Geometry check sheet. Reference: the model listing, model coordinates, mm. Face numbers are marked on the shaded views. A direction names the side the tool comes from. Give positions to 0.01 mm unless a question says otherwise; leave off trailing zeros. Order: outer loops, then holes, each group sorted by start corner. A loop starts at its lowest first (then second) coordinate and runs counter-clockwise, first axis right, second up. Notation, with made-up numbers: M 64,81.25 L 71,81.25 A25 cw 71,94.25 Z; hole C 29.5,-35.5 d2. An arc over 180 degrees is marked long. Answer as a JSON object with one key per item and string values. Group by question number.
Autodesk Inventor part; units mm, degrees
ref_plane "YZ Plane" through (0, 0, 0) normal (1, 0, 0) x (0, 1, 0)
ref_plane "XZ Plane" through (0, 0, 0) normal (0, 1, 0) x (-1, 0, 0)
ref_plane "XY Plane" through (0, 0, 0) normal (0, 0, 1) x (1, 0, 0)
ref_plane "РабПлоскость1" through (-45, 39.0097, 0) normal (-0.9659258, 0, 0.258819) x (0, -1, 0)
sketch "Эскиз1" plane through (-45, 39.0097, 0) normal (-0.9659258, 0, 0.258819) x (0, -1, 0)
  line L0 (0, 0) -> (78.0194, 0)
  line L1 (0.0194, 85.4597) -> (78.0194, 85.4597)
  line L2 (78.0194, 68.8953) -> (78.0194, 85.4597)
  line L3 (-2.9723, 68.8953) -> (78.0194, 68.8953)
  line L4 (-2.9723, 68.8953) -> (-2.9723, 74.9718)
  ellipse E0 centre (-19.9806, 77.6951) end of major axis (0.0194, 77.6951) minor radius 5.1764 (-2.9723, 74.9718) -> (0.0194, 77.6951) ccw
  line L5 (0.0194, 80.2833) -> (0.0194, 77.6951)
  line L6 (0.0194, 80.2833) -> (0.0194, 85.4597)
  line L7 (0, 0) -> (78.0194, 0)
  line L8 (78.0194, 0) -> (78.0194, 90.4597)
  line L9 (78.0194, 90.4597) -> (0, 90.4597)
  line L10 (0, 90.4597) -> (0, 0)
  point P0 (39.0097, 11.6469)
  dimension "d1" = 5
extrude "Выдавливание1" add sketch "Эскиз1" against normal blind 2 contours L10 L3 L8 L0 | L10 E0 L5 L6 L1 L2 L3 | L10 L9 L8 L1 L6 L5 E0
sketch "Эскиз2" plane through (-43.0681, 39.0097, -0.5176) normal (0.9659258, 0, -0.258819) x (-0.258819, 0, -0.9659258)
  line L0 (0, 0) -> (0, -78.0194)
  line L1 (0, -78.0194) -> (-90.4597, -78.0194)
  line L2 (-90.4597, -78.0194) -> (-90.4597, -76.0194)
  line L3 (-90.4597, -76.0194) -> (0, -76.0194)
  line L4 (0, -76.0194) -> (0, -78.0194)
  line L5 (0, 0) -> (-90.4597, 0)
  line L6 (-90.4597, 0) -> (-90.4597, -2)
  line L7 (-90.4597, -2) -> (0, -2)
  line L8 (0, -2) -> (0, 0)
  line L9 (-90.4597, -78.0194) -> (-90.4597, 0)
  line L10 (-90.4597, -76.0194) -> (-88.4597, -76.0194)
  line L11 (-88.4597, -76.0194) -> (-88.4597, -2)
  line L12 (-88.4597, -2) -> (-90.4597, -2)
  line L13 (-90.4597, -2) -> (-90.4597, -76.0194)
  line L14 (-66.4597, -76.0194) -> (-68.4597, -76.0194)
  line L15 (-68.4597, -76.0194) -> (-68.4597, -2)
  line L16 (-68.4597, -2) -> (-66.4597, -2)
  line L17 (-66.4597, -2) -> (-66.4597, -76.0194)
  point P0 (-11.6469, -39.0097)
  point P1 (-90.4597, -1)
  point P2 (-90.4597, -77.0194)
  point P3 (-89.4597, -2)
  point P4 (-90.4597, -76.0194)
  point P5 (0, -76.0194)
  point P6 (-66.4597, -2)
  point P7 (0, -2)
  point P8 (-90.4597, -2)
  point P9 (-88.4597, -76.0194)
  point P10 (-88.4597, -2)
  dimension "d4" = 2
  dimension "d5" = 2
  dimension "d6" = 2
  dimension "d7" = 2
  dimension "d8" = 20
extrude "Выдавливание2" add sketch "Эскиз2" along normal blind 2 contours L0 L7 L6 L5 | L0 L1 L2 L3 | L17 L3 L15 L7 | L7 L11 L3 L9
ref_plane "РабПлоскость2" through (-23.4176, 37.0097, 65.0917) normal (0.258819, 0, 0.9659258) x (0, -1, 0)
sketch "Эскиз3" plane through (-23.4176, 37.0097, 65.0917) normal (0.258819, 0, 0.9659258) x (0, -1, 0)
  line L0 (-2, 0) -> (76.0194, 0)
  point P0 (37.0097, 39.4667)
sketch "Эскиз4" plane through (-23.4176, 37.0097, 65.0917) normal (0.258819, 0, 0.9659258) x (0, -1, 0)
  line L0 (76.0194, 0) -> (-2, 0)
  line L1 (-2, 0) -> (-2, 15)
  line L2 (-2, 15) -> (76.0194, 15)
  line L3 (76.0194, 15) -> (76.0194, 0)
  point P0 (37.0097, 39.4667)
  dimension "d12" = 15
extrude "Выдавливание3" add sketch "Эскиз4" along normal blind 2
properties part number "ДИ 00.00.09"
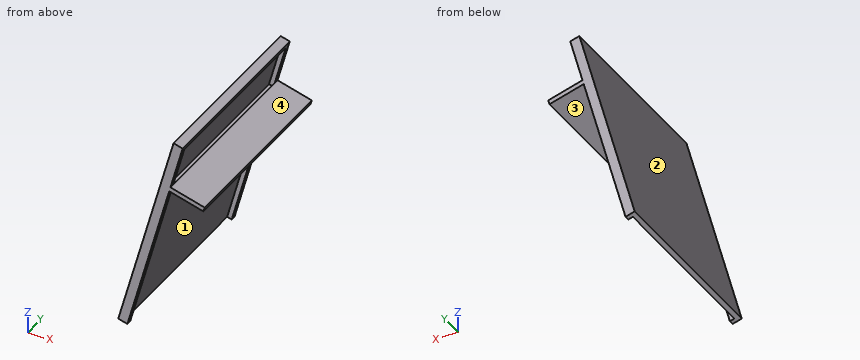
1. Cross-section at C-C (z = 70.5). Record the cut outline in (x, y), and give its area (3 significant figures).
2. Release check for a two-part mould opening along Y. For the marked faces 1 and 2 record: released by +Y, released by -Y, zero draft, split by the parting line, or undercut.
3. Thickness scan on line 1 along X through (y, z) = (26.5, 8.5); line 2 along X through (y, z) = (-6, 68); line 3 along Z through (x, y) = (-11.5, 17.5). Record the ranges inside material, lowest first. Write a range as [from, to].
4. Cross-section at D-D (x = -15.5). Record the cut outline in (y, z).
5. Cross-section at B-B (x = -32.5). Record the cut outline in (y, z).
6. Depth check by flat-ended pin: pin 1 (3 mm diameter, centred on y = -12.5, z = 36.5, fed in from -X); pin 2 (5 mm diameter, centred on y = 23, z = 58.5, fed in from -X); pin 3 (1 mm diameter, centred on y = 18.5, z = 32.5, fed in from +X). Enter the tip coordinate at first touch or a pass-through.
7. Access from +Z, -Z, +X, -X, +Y, -Y to the whole of each face (thin tool, end or side, straight path). Record for the marked faces 3 and 4.
Report:
{
 "1": {"outline": "M -26.11,-39.01 L -21.97,-39.01 L -21.97,-37.01 L -24.04,-37.01 L -24.04,37.01 L -21.97,37.01 L -21.97,39.01 L -26.11,39.01 Z", "area": "170 mm2"},
 "2": {"face 1": "undercut", "face 2": "zero draft"},
 "3": {"line 1": "x = [-42.72, -40.65]", "line 2": "x = [-26.78, -24.71]", "line 3": "z = [61.9, 63.97]"},
 "4": {"outline": "M -39.01,62.97 L 39.01,62.97 L 39.01,65.04 L -39.01,65.04 Z"},
 "5": {"outline": "M -39.01,31.2 L -37.01,31.2 L -37.01,38.92 L 37.01,38.92 L 37.01,31.2 L 39.01,31.2 L 39.01,46.65 L -39.01,46.65 Z"},
 "6": {"pin 1": "stops at x = -35.62", "pin 2": "stops at x = -29.99", "pin 3": "stops at x = -34.09"},
 "7": {"face 3": "-Z, +Y, -Y", "face 4": "+X, +Y, -Y"}
}
